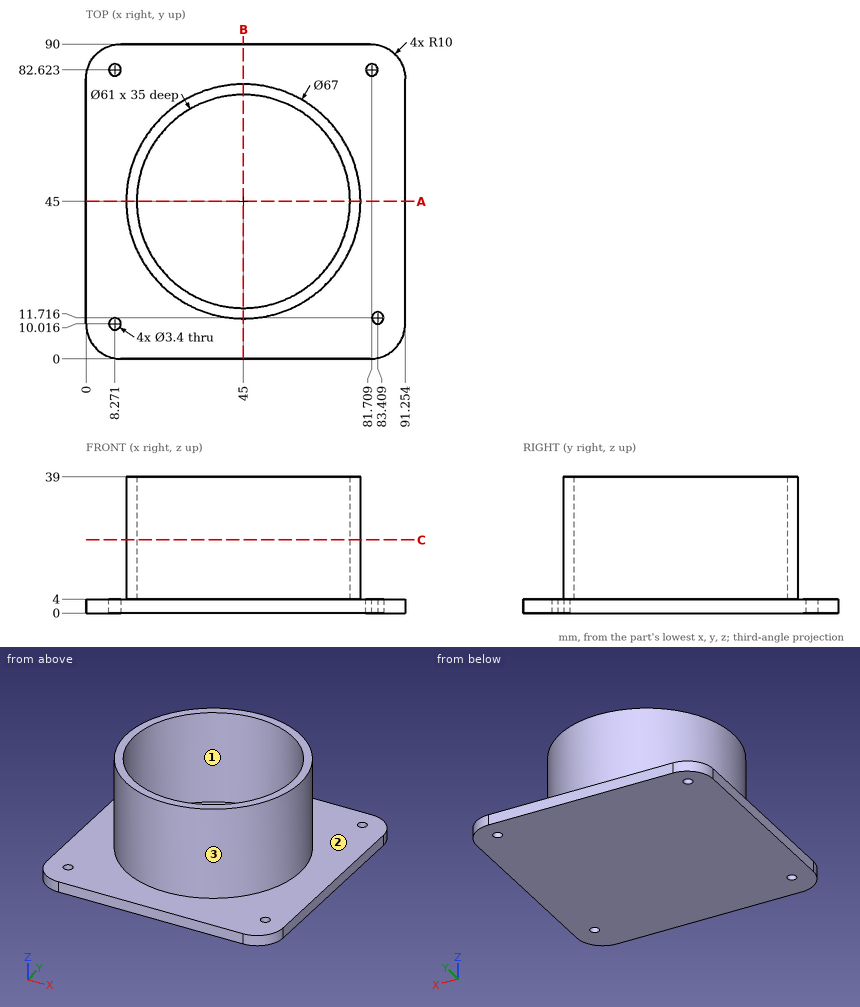
Input: dimensioned drawing with shaded views. Units: mm. Origin: part minimum x, y, z. Coordinates: 2 decimals unless noted, no trailing zeros. Order: outer loops, then holes, each group sorted by start corner. A loop starts at its lowest first (then second) coordinate and runs counter-clockwise, first axis right, second up.
(1) Section query A-A (y = 45). Return the cut outline in (x, z), plus the area to 3 significant figures.
(2) Section query C-C (z = 21). Return the cut outline in (x, y).
(3) Section query B-B (x = 45). Return the cut outline in (y, z).
(4) Draft query along Y for the marked faces 1, 2 and 3. Return one class per face: pulls with the +Y half, pulls with the -Y half, needs draft (parallel to the pull), parting line crosses it, or undercut.
(5) First-contact query: pin 1 (10 mm diameter, centred on x = 66.5, z = 12.5, fed in from -Y) (1 decimal); pin 2 (4.5 mm diameter, centred on x = 81.71, y = 82.62, fed in from -Z); pin 3 (8 mm diameter, centred on x = 18.5, y = 76.5, fed in from +Z); pin 4 (8 mm diameter, centred on x = 49, z = 11, fed in from +Y). Flat tips, straight axial feed; report the tip coordinate or a pass-through.
(6) Material intervals for probe 1 along X at (y, z) = (46, 9.5) (1 decimal); probe 2 along Z at (x, y) = (82, 47), sorted ascending.
Solution:
1. outline: (0, 0) - (91.25, 0) - (91.25, 4) - (78.5, 4) - (78.5, 39) - (75.5, 39) - (75.5, 4) - (14.5, 4) - (14.5, 39) - (11.5, 39) - (11.5, 4) - (0, 4) - close
1. area: 575 mm2
2. outline: circle Ø67 at (45, 45); hole circle Ø61 at (45, 45)
3. outline: (0, 0) - (90, 0) - (90, 4) - (78.5, 4) - (78.5, 39) - (75.5, 39) - (75.5, 4) - (14.5, 4) - (14.5, 39) - (11.5, 39) - (11.5, 4) - (0, 4) - close
4. face 1: undercut
4. face 2: needs draft
4. face 3: parting line crosses it
5. pin 1: stops at y = 15.8
5. pin 2: stops at z = 0
5. pin 3: stops at z = 4
5. pin 4: stops at y = 78.5
6. probe 1: x = 11.5 to 14.5, 75.5 to 78.5
6. probe 2: z = 0 to 4
